The listing builds one solid part. Answer for the finished solid, in the listing's coordinates (mm). A direction names the side the tool comes from. Give positions to 0.01 mm unless a question says otherwise; leave off trailing zeros. Write each loop counter-clockwise with the first axis right and the second up, starting at its lowest first coordinate (ties: lowest second). Pieces come first, ordered by that corner, then holes. Notation, with made-up numbers: (69.25, -35.5) - (116.25, -35.5) arc R29 cw to (116.25, -1.5) - close; hole circle Ø4 at (49, 15). An arc over 180 degrees is marked (long way). Write each question's results on one line, items separated by ' | '. Start each with the question number.
Q1. Section B-B (x = 68.5) is taken. Determine the outline of the cut face in (y, z), plus the area to 3 significant figures.
Q2. Section C-C (z = 2.65) is taken. Determine the outline of the cut face in (x, y).
Q3. Section A-A (y = 19) is taken. Determine the outline of the cut face in (x, z).
Q4. For faces 5 (the face through (17, 35, 3)), 6 (the face through (55, 48, 1)), 7 (the face through (48, 35, 0)), 8 (the face through (15.1, 35, 1)), 9 (the face through (79.7, 35, 3)), determine the directions among +Z, -Z, +X, -X, +Y, -Y from which every point of the face is accessible in a straight line to the end or side of a thin tool.
Q5. Flat-ended cylindrical pins translate along their axes: pin 1 Ø6 at (x, y) = (74, 48.5) entering from +Z; pin 2 Ø1.9 at (y, z) = (39.5, 3) entering from -X; pin 3 Ø1.9 at (y, z) = (31, 3) entering from +X. Find the tip coordinate at first contact, or state that the pin passes through.
Q6. For a pull along X with two mould halves and no side action, classify faces 1 (the face through (81.6, 35, 1)), 2 (the face through (79.35, 30.5, 1.9)), 3 (the face through (48.784, 39.146, 2.521)), 4 (the face through (49, 6.25, 1)) as pulls with the +X half, pulls with the -X half, needs draft (parallel to the pull), parting line crosses it, or undercut.
Q7. Find the intervals of material crossed by probe 1 along Y at (x, z) = (49, 1.15); probe 2 along Y at (x, z) = (25.5, 1.35); probe 3 along X at (y, z) = (38.5, 2.75), in increasing order.
Autodesk Fusion 360 part; units mm, degrees
sketch "Schizzo1" plane through (0, 0, 0) normal (0, 0, 1) x (1, 0, 0)
  line L0 (15, 63.85) -> (81.7, 63.85) construction
  line L1 (81.7, 63.85) -> (81.7, 6.15) construction
  line L2 (81.7, 6.15) -> (15, 6.15) construction
  line L3 (15, 6.15) -> (15, 63.85) construction
  line L4 (15, 35) -> (81.7, 35) construction
  line L5 (48.35, 63.85) -> (48.35, 6.15) construction
  line L6 (81.6, 6.25) -> (15.1, 6.25)
  line L7 (15.1, 6.25) -> (15.1, 63.75)
  line L8 (15.1, 63.75) -> (81.6, 63.75)
  line L9 (81.6, 63.75) -> (81.6, 6.25)
  line L10 (79.7, 8.15) -> (17, 8.15)
  line L11 (17, 8.15) -> (17, 61.85)
  line L12 (17, 61.85) -> (79.7, 61.85)
  line L13 (79.7, 61.85) -> (79.7, 8.15)
  line L14 (15.1, 40) -> (81.7, 40)
  line L15 (15.1, 30) -> (81.7, 30)
  line L16 (17, 61.85) -> (45, 61.85)
  line L17 (45, 61.85) -> (45, 51.85)
  line L18 (45, 51.85) -> (17, 51.85)
  line L19 (17, 51.85) -> (17, 61.85)
  dimension "d1" = 66.7
  dimension "d2" = 57.7
  dimension "d3" = 0.1
  dimension "d4" = 2
  dimension "d9" = 10
  dimension "d18" = 28
  dimension "d19" = 10
extrude "Estrusione1" add sketch "Schizzo1" along normal blind 1 contours L11 L13 L14 L15 | L10 L11 L13 L15 | L11 L12 L13 L14 L17 L18
extrude "Estrusione2" add sketch "Schizzo1" along normal blind 2 contours L6 L7 L9 L10 L11 L13 L15 | L9 L13 L14 L15 | L7 L11 L14 L15 | L7 L8 L9 L11 L12 L13 L14 L16 L19
fillet "Raccordo1" radius 2 4 edges at (81.6, 6.25, 1) (15.1, 6.25, 1) (81.6, 63.75, 1) (15.1, 63.75, 1)
extrude "Estrusione3" add sketch "Schizzo1" along normal blind 4 contours L11 L13 L14 L15
ref_plane "Piano di lavoro1" through (48.35, 35, 0) normal (-1, 0, 0) x (0, -1, 0)
sketch "Schizzo2" plane through (48.35, 0, 0) normal (-1, 0, 0) x (0, -1, 0)
  line L0 (-30, 4) -> (-40, 4) construction
  line L1 (-40, 4) -> (-40, 1) construction
  line L2 (-40, 1) -> (-30, 1) construction
  line L3 (-30, 1) -> (-30, 4) construction
  line L4 (-30, 1) -> (-30, 4)
  line L5 (-30, 4) -> (-31.7321, 1)
  line L6 (-31.7321, 1) -> (-30, 1)
  line L7 (-35, 4) -> (-35, 1) construction
  line L8 (-40, 4) -> (-38.2679, 1)
  line L9 (-40, 1) -> (-40, 4) construction
  line L10 (-38.2679, 1) -> (-40, 1)
  line L11 (-40, 1) -> (-40, 4)
  point P0 (-40, 1)
  point P1 (-30, 4)
  dimension "d15" = 30
extrude "Estrusione4" cut sketch "Schizzo2" along normal mid plane 62
Answers below:
1) outline: (6.25, 0) - (63.75, 0) - (63.75, 2) - (61.85, 2) - (61.85, 1) - (38.27, 1) - (40, 4) - (30, 4) - (31.73, 1) - (8.15, 1) - (8.15, 2) - (6.25, 2) - close | area: 86.1 mm2
2) outline: (17, 30) - (17.35, 30) - (17.35, 30.78) - (79.35, 30.78) - (79.35, 30) - (79.7, 30) - (79.7, 40) - (79.35, 40) - (79.35, 39.22) - (17.35, 39.22) - (17.35, 40) - (17, 40) - close
3) outline: (15.1, 0) - (81.6, 0) - (81.6, 2) - (79.7, 2) - (79.7, 1) - (17, 1) - (17, 2) - (15.1, 2) - close
4) face 5: +Z, -X, +Y, -Y | face 6: none | face 7: -Z, +X, -X, +Y, -Y | face 8: +Z, -Z, -X, +Y, -Y | face 9: +Z, +X, +Y, -Y
5) pin 1: stops at z = 1 | pin 2: stops at x = 17 | pin 3: stops at x = 79.7
6) face 1: pulls with the +X half | face 2: undercut | face 3: undercut | face 4: needs draft
7) probe 1: y = 6.25 to 8.15, 31.65 to 38.35, 61.85 to 63.75 | probe 2: y = 6.25 to 8.15, 31.53 to 38.47, 61.85 to 63.75 | probe 3: x = 17 to 79.7
